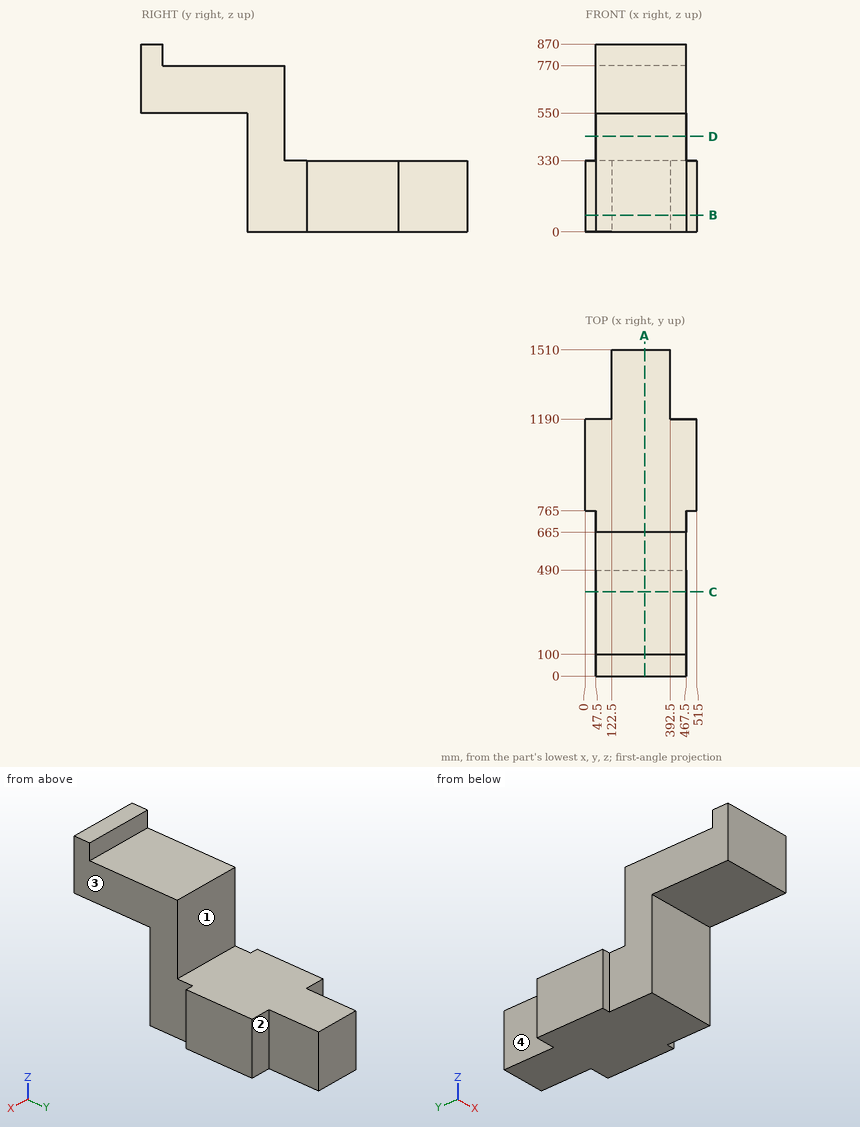
Check sheet for the drawn part. Datum: minimum x, y, z corner. Units: mm. A direction names the side the tool comes from. Give positions to 0.01 mm unless a question says otherwise; leave off trailing zeros. Order: outer loops, then holes, each group sorted by start corner. A loop starts at its lowest first (then second) coordinate and runs counter-clockwise, first axis right, second up. Notation, with made-up numbers: (51.25, 74) -> (72.25, 74) arc R20 cw to (72.25, 101) -> close; hole circle Ø8 at (-12, 45). An arc over 180 degrees is marked (long way). One line per item, written item: value.
(1) Sectioned sample at B-B on z = 78. Record the cut outline in (x, y), then the cut area to 3 significant figures.
Final values:
outline: (0, 765) -> (47.5, 765) -> (47.5, 490) -> (467.5, 490) -> (467.5, 765) -> (515, 765) -> (515, 1190) -> (392.5, 1190) -> (392.5, 1510) -> (122.5, 1510) -> (122.5, 1190) -> (0, 1190) -> close
area: 421,000 mm^2
(2) Sectioned sample at D-D on z = 442. Record the cut outline in (x, y).
Final values:
outline: (47.5, 490) -> (467.5, 490) -> (467.5, 665) -> (47.5, 665) -> close
(3) Scan lines: line 1 along Z through (x, y) = (52, 395.5); line 2 along Y through (x, z) = (269.5, 300); line 3 along Z through (x, y) = (25.5, 868). Record each from-to range of solid material in increasing order. Write a range as [from, to].
Final values:
line 1: [550, 770]
line 2: [490, 1510]
line 3: [0, 330]
(4) Gauge pin test, flat ends, axial feed: pin 1 (1.5 mm diameter, centred on x = 131.5, y = 1210.5, fed in from -Z); pin 2 (1 mm diameter, centred on x = 269, y = 163, fed in from +Z); pin 3 (6 mm diameter, centred on x = 244, z = 398.5, fed in from -Y); pin 4 (5 mm diameter, centred on x = 460, y = 273, fed in from -Z). Record the tip position at first contact, or that the pin passes through.
Final values:
pin 1: z = 0
pin 2: z = 770
pin 3: y = 490
pin 4: z = 550
(5) Sectioned sample at C-C on y = 389. Record the cut outline in (x, z), then the cut area to 3 significant figures.
Final values:
outline: (47.5, 550) -> (467.5, 550) -> (467.5, 770) -> (47.5, 770) -> close
area: 92,400 mm^2
(6) Sectioned sample at A-A on x = 274. Record the cut outline in (y, z).
Final values:
outline: (0, 550) -> (490, 550) -> (490, 0) -> (1510, 0) -> (1510, 330) -> (665, 330) -> (665, 770) -> (100, 770) -> (100, 870) -> (0, 870) -> close
(7) Tool access check on the marked faces 1, 2, 3 and 4. Record the directions out of +Z, -Z, +X, -X, +Y, -Y that give a thin tool (end or side, any length) a straight path to the whole face; none if there is none.
Final values:
face 1: +Z, +X, -X, +Y
face 2: +Z, -Z, +X, +Y
face 3: +Z, -Z, +X, -Y
face 4: +Z, -Z, -X, +Y
